For this review, take the finished solid that the model builds, in its own axes (mm). Round coordinates to 2 decimals unless told otherwise and drop trailing zeros. Order: outer loops, then holes, each group sorted by start corner. A loop starts at its lowest first (then second) coordinate and runs counter-clockwise, first axis right, second up. Notation, with made-up numbers: (-22.75, 73.25) -> (32.25, 73.25) arc R21 cw to (32.25, 92.25) -> close; hole circle Ø5 at (-25, 13.25). An arc over 180 degrees is marked (long way). Put each result on its own line as item: value. Start each with the question number.
```python
from build123d import *

# Parameters (mm, degrees)
SKETCH1_W           = 38.1
SKETCH1_H           = 6.35
BOSS_EXTRUDE1_DEPTH = 3.175
SKETCH2_R           = 1.5748
CUT_EXTRUDE1_DEPTH  = 4.175
LPATTERN1_COUNT     = 6
LPATTERN1_PITCH     = 6.35


with BuildPart() as part:
    # Sketch1 → Boss-Extrude1 (new body)
    with BuildSketch(Plane(origin=(0, 0, 0), x_dir=(1, 0, 0), z_dir=(0, 1, 0))):
        Rectangle(SKETCH1_W, SKETCH1_H)
    extrude(amount=BOSS_EXTRUDE1_DEPTH)

    # Sketch2 → Cut-Extrude1 (cut, through all)
    with BuildSketch(Plane(origin=(0, 3.175, 0), x_dir=(1, 0, 0), z_dir=(0, 1, 0))):
        with Locations((15.875, 0)):
            Circle(SKETCH2_R)
    cut_extrude1 = extrude(amount=-CUT_EXTRUDE1_DEPTH, mode=Mode.SUBTRACT)

    # LPattern1: Cut-Extrude1 ×6
    with Locations(*[(-i * LPATTERN1_PITCH, 0, 0) for i in range(1, LPATTERN1_COUNT)]):
        add(cut_extrude1, mode=Mode.SUBTRACT)


solid = part.part
```
Item 1: Mouldability with a two-part tool opening along Z and no side actions: class faces 1 (the face through (7.95, 1.61, -0.07)), 2 (the face through (0, 2, -3.175)), 3 (the face through (19.05, 2, 0)) as +Z half, -Z half, draft (parallel to the pull), parting line (faces both ways), or undercut.
Item 2: Consider section B-B, the plane y = 0.65. Write out the cut boundary in (x, z) (3 decimals).
Item 3: For L1, parallel to Z at x = -17, y = 2.2 (3 decimals); L2, parallel to Z at x = 9, y = 0.45 (3 decimals), list the stretches that pass through material, from the lowest coordinate up.
Item 4: Consider section C-C, the plane x = 10.5. Write out the cut boundary in (y, z) (3 decimals), plus the area to 3 significant figures.
Item 5: Consider section D-D, the plane x = -9.5. Write out the cut boundary in (y, z) (3 decimals).
Item 6: Consider section A-A, the plane z = 0. Write out the cut boundary in (x, y) (3 decimals).
Evaluation:
1. face 1: undercut
1. face 2: -Z half
1. face 3: draft
2. outline: (-19.05, -3.175) -> (19.05, -3.175) -> (19.05, 3.175) -> (-19.05, 3.175) -> close; hole circle Ø3.15 at (-15.875, 0); hole circle Ø3.15 at (-9.525, 0); hole circle Ø3.15 at (-3.175, 0); hole circle Ø3.15 at (3.175, 0); hole circle Ø3.15 at (9.525, 0); hole circle Ø3.15 at (15.875, 0)
3. L1: z = -3.175 to -1.102, 1.102 to 3.175
3. L2: z = -3.175 to -1.485, 1.485 to 3.175
4. outline: (0, -3.175) -> (3.175, -3.175) -> (3.175, -1.237) -> (0, -1.237) -> close; (0, 1.237) -> (3.175, 1.237) -> (3.175, 3.175) -> (0, 3.175) -> close
4. area: 12.3 mm^2
5. outline: (0, -3.175) -> (3.175, -3.175) -> (3.175, -1.575) -> (0, -1.575) -> close; (0, 1.575) -> (3.175, 1.575) -> (3.175, 3.175) -> (0, 3.175) -> close
6. outline: (-19.05, 0) -> (-17.45, 0) -> (-17.45, 3.175) -> (-19.05, 3.175) -> close; (-14.3, 0) -> (-11.1, 0) -> (-11.1, 3.175) -> (-14.3, 3.175) -> close; (-7.95, 0) -> (-4.75, 0) -> (-4.75, 3.175) -> (-7.95, 3.175) -> close; (-1.6, 0) -> (1.6, 0) -> (1.6, 3.175) -> (-1.6, 3.175) -> close; (4.75, 0) -> (7.95, 0) -> (7.95, 3.175) -> (4.75, 3.175) -> close; (11.1, 0) -> (14.3, 0) -> (14.3, 3.175) -> (11.1, 3.175) -> close; (17.45, 0) -> (19.05, 0) -> (19.05, 3.175) -> (17.45, 3.175) -> close
